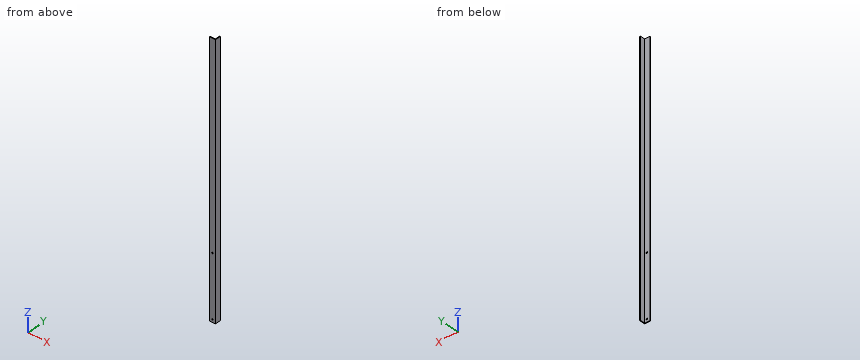
```python
from build123d import *

# Parameters (mm, degrees)
F1_DEPTH = 1727.2
F2_R     = 4.7625
F3_DEPTH = 38.101
F4_R     = 4.7625
F5_DEPTH = 38.101


with BuildPart() as f1:
    # F0 (on Top) → F1 (new body)
    with BuildSketch(Plane.XY):
        Polygon((0, 4.7625), (0, 0), (38.1, 0), (38.1, 38.1), (33.3375, 38.1), (33.3375, 4.7625), align=None)
    extrude(amount=F1_DEPTH)

    # F2 (on face) → F3 (cut, through all)
    with BuildSketch(Plane.XZ):
        with Locations((19.05, 19.05)):
            Circle(F2_R)
    extrude(amount=-F3_DEPTH, mode=Mode.SUBTRACT)

    # F4 (on face) → F5 (cut, through all)
    with BuildSketch(Plane.XZ):
        with Locations((19.05, 422.275)):
            Circle(F4_R)
    extrude(amount=-F5_DEPTH, mode=Mode.SUBTRACT)


solid = f1.part
```
Model file for the job. Use its own axes, mm. Coordinates: 2 decimals unless noted, no trailing zeros. Write each loop counter-clockwise with the first axis right and the second up, starting at its lowest first coordinate (ties: lowest second). Pieces come first, ordered by that corner, then holes. Notation, with made-up numbers: (-5, -35.5) - (46, -35.5) arc R21 ccw to (46, -8.5) - close; hole circle Ø5 at (61.5, 51.25). An arc over 180 degrees is marked (long way). Use a Markdown table: item, result. Add a question column.
Item 1: Band-saw the part on B-B, the plane x = 6. Write the cut outline in (y, z).
Item 2: Drill centre lines: line 1 along Z through (x, y) = (19.05, 1.6); line 2 along Y through (x, z) = (12, 1099.5); line 3 along X through (y, z) = (19, 1205). Where is each one in solid material? Low to high.
Item 3: Band-saw the part on C-C, the plane y = 12. Write the cut outline in (x, z), and give its area (3 significant figures).
Item 4: Band-saw the part on A-A, the plane z = 1161.5. Write the cut outline in (x, y).
Item 5: Drop flat-ended pins along their axis: pin 1 (16.5 mm diameter, centred on x = 22, z = 601.5, fed in from +Y); pin 2 (16.5 mm diameter, centred on y = 16, z = 536.5, fed in from -X). Give the stop position or say it passes through.
A:
| question | item | result |
|---|---|---|
| 1 | outline | (0, 0) - (4.76, 0) - (4.76, 1727.2) - (0, 1727.2) - close |
| 2 | line 1 | z = 0 to 14.29, 23.81 to 417.51, 427.04 to 1727.2 |
| 2 | line 2 | y = 0 to 4.76 |
| 2 | line 3 | x = 33.34 to 38.1 |
| 3 | outline | (33.34, 0) - (38.1, 0) - (38.1, 1727.2) - (33.34, 1727.2) - close |
| 3 | area | 8,230 mm² |
| 4 | outline | (0, 0) - (38.1, 0) - (38.1, 38.1) - (33.34, 38.1) - (33.34, 4.76) - (0, 4.76) - close |
| 5 | pin 1 | stops at y = 4.76 |
| 5 | pin 2 | stops at x = 33.34 |
